Read the model definition and answer for the solid it produces. Units are mm, in the model's axes. A direction names the side the tool comes from. Round coordinates to 2 decimals unless told otherwise and drop trailing zeros. Order: outer loops, then holes, each group sorted by start corner. A loop starts at its lowest first (then second) coordinate and runs counter-clockwise, first axis right, second up. Notation, with made-up numbers: (44, -12.5) -> (72, -12.5) arc R16 cw to (72, 15.5) -> close; hole circle Ø2 at (20, -4). An arc over 180 degrees is marked (long way). One line per item, written item: value. Start each with the question number.
1. For faces 1 (the face through (21.25, 0.08, 0.51)), 2 (the face through (-11, -22, 1)), determine the directions among +Z, -Z, +X, -X, +Y, -Y from which every point of the face is accessible in a straight line to the end or side of a thin tool.
2. Section C-C (y = -15.5) is taken. State how many separate pieces and enclosed holes the cut face has, then the cut area to 3 significant figures.
3. Section B-B (z = 4.25) is taken. Give the vertices of the cut face in (x, y).
4. Flat-ended cylindrical pins translate along their axes: pin 1 Ø1.5 at (x, y) = (22, 0.5) entering from +Z; pin 2 Ø2 at (y, z) = (-15.5, 3.5) entering from +X; pin 3 Ø2 at (x, y) = (16.26, -16.26) entering from +Z; pin 4 Ø2 at (y, z) = (20.5, 0.5) entering from -X. Find the tip coordinate at first contact, or state that the pin passes through.
5. Section A-A (y = 3.5) is taken. Give the vertices of the cut face in (x, z).
6. Consider line 1 (Y direction, x = 0, z = 1.35); line 2 (Y direction, x = -3.5, z = 4.6); line 3 (X direction, y = -18.5, z = 3.8). Determine where each line is inside the solid, lowest interval first.
7. The mould has two halves that part along X. Classify faces 3 (the face through (18.1, -9, 5)), 4 (the face through (-2, 22, 1)): released by +X, released by -X, zero draft, split by the parting line, or undercut.
from build123d import *

# Parameters (mm, degrees)
F0_R     = 26
F0_R_2   = 20
F1_DEPTH = 5
F2_R     = 25.5
F2_R_2   = 20.5
F3_DEPTH = 2.5
F4_R     = 2.5
F5_DEPTH = 1.5
F6_R     = 1.75
F7_DEPTH = 2.501


with BuildPart() as f1:
    # F0 (on Top) → F1 (new body)
    with BuildSketch(Plane.XY):
        Circle(F0_R)
        Circle(F0_R_2, mode=Mode.SUBTRACT)
    extrude(amount=F1_DEPTH)

    # F2 (on face) → F3 (cut)
    with BuildSketch(Plane.XY.offset(5)):
        Circle(F2_R)
        Circle(F2_R_2, mode=Mode.SUBTRACT)
    extrude(amount=-F3_DEPTH, mode=Mode.SUBTRACT)

    # F4 (on face) → F5 (cut)
    with BuildSketch(Plane.XY.offset(2.5)):
        with Locations((23, 0)):
            Circle(F4_R)
        with Locations((21.249229, -8.801719)):
            Circle(F4_R)
        with Locations((16.263456, -16.263456)):
            Circle(F4_R)
        with Locations((8.801719, -21.249229)):
            Circle(F4_R)
        with Locations((0, -23)):
            Circle(F4_R)
        with Locations((-8.801719, -21.249229)):
            Circle(F4_R)
        with Locations((-16.263456, -16.263456)):
            Circle(F4_R)
        with Locations((-21.249229, -8.801719)):
            Circle(F4_R)
        with Locations((-23, 0)):
            Circle(F4_R)
        with Locations((-21.249229, 8.801719)):
            Circle(F4_R)
        with Locations((-16.263456, 16.263456)):
            Circle(F4_R)
        with Locations((-8.801719, 21.249229)):
            Circle(F4_R)
        with Locations((0, 23)):
            Circle(F4_R)
        with Locations((8.801719, 21.249229)):
            Circle(F4_R)
        with Locations((16.263456, 16.263456)):
            Circle(F4_R)
        with Locations((21.249229, 8.801719)):
            Circle(F4_R)
    extrude(amount=-F5_DEPTH, mode=Mode.SUBTRACT)

    # F6 (on face) → F7 (cut, through all)
    with BuildSketch(Plane.XY.offset(2.5)):
        with Locations((23, 0)):
            Circle(F6_R)
        with Locations((21.249229, 8.801719)):
            Circle(F6_R)
        with Locations((16.263456, 16.263456)):
            Circle(F6_R)
        with Locations((8.801719, 21.249229)):
            Circle(F6_R)
        with Locations((0, 23)):
            Circle(F6_R)
        with Locations((-8.801719, 21.249229)):
            Circle(F6_R)
        with Locations((-16.263456, 16.263456)):
            Circle(F6_R)
        with Locations((-21.249229, 8.801719)):
            Circle(F6_R)
        with Locations((-23, 0)):
            Circle(F6_R)
        with Locations((-21.249229, -8.801719)):
            Circle(F6_R)
        with Locations((-16.263456, -16.263456)):
            Circle(F6_R)
        with Locations((-8.801719, -21.249229)):
            Circle(F6_R)
        with Locations((0, -23)):
            Circle(F6_R)
        with Locations((8.801719, -21.249229)):
            Circle(F6_R)
        with Locations((16.263456, -16.263456)):
            Circle(F6_R)
        with Locations((21.249229, -8.801719)):
            Circle(F6_R)
    extrude(amount=-F7_DEPTH, mode=Mode.SUBTRACT)


solid = f1.part
Answer:
1. face 1: +Z, -Z
1. face 2: +Z
2. separate pieces: 4
2. enclosed holes: 0
2. area: 27.6 mm^2
3. outline: circle Ø52 at (0, 0); circle Ø41 at (0, 0); hole circle Ø51 at (0, 0); hole circle Ø40 at (0, 0)
4. pin 1: z = 1
4. pin 2: x = 21.58
4. pin 3: through
4. pin 4: x = -17.2
5. outline: (-25.76, 0) -> (-19.69, 0) -> (-19.69, 5) -> (-20.2, 5) -> (-20.2, 2.5) -> (-25.26, 2.5) -> (-25.26, 5) -> (-25.76, 5) -> close; (19.69, 0) -> (25.76, 0) -> (25.76, 5) -> (25.26, 5) -> (25.26, 2.5) -> (20.2, 2.5) -> (20.2, 5) -> (19.69, 5) -> close
6. line 1: -26 to -25.5, -20.5 to -20, 20 to 20.5, 25.5 to 26
6. line 2: -25.76 to -25.26, -20.2 to -19.69, 19.69 to 20.2, 25.26 to 25.76
6. line 3: -18.27 to -17.55, -8.83 to -7.6, 7.6 to 8.83, 17.55 to 18.27
7. face 3: zero draft
7. face 4: undercut
